Geometry: final body of the model. Coordinates: model frame, mm. Give positions to 0.01 mm unless a question says otherwise; leave off trailing zeros. Write each loop counter-clockwise with the first axis right and the second up, starting at its lowest first coordinate (ties: lowest second). Pieces come first, ordered by that corner, then holes.
Q1. Cut plane D-D on x = 14. Return the cut outline in (y, z) (3 decimals), plus the area to 3 significant figures.
Q2. Cut plane C-C on y = 15. Return the cut outline in (x, z) (3 decimals).
Q3. Line query: L1, parallel to X at y = 25, z = 0.8; L2, parallel to Y at x = 6, z = 1.7; L3, parallel to Z at x = 16.5, y = 17. Output: solid intervals per line, ascending.
Q4. Cut plane B-B on x = 6. Return the cut outline in (y, z).
Q5. Cut plane A-A on y = 5. Return the cut outline in (x, z).
Q6. Pin query (flat end, axial travel): pin 1 (4 mm diameter, centred on y = 20, z = -16, fed in from +X); pin 2 (10 mm diameter, centred on x = 16, z = -10, fed in from -Y) (3 decimals); pin 3 (2 mm diameter, centred on y = 14.5, z = -11.5, fed in from +X) (3 decimals); pin 4 (1 mm diameter, centred on x = 7.5, y = 22, fed in from -Z). Return the tip coordinate at first contact, or that it passes through.
Q7. Draft query along Y for faces 1 (the face through (23.5, 4.93, 1.52)), 2 (the face through (6.195, 23.513, 1.521)), 3 (the face through (16.305, 15.956, -23.91)), 4 (the face through (0, 15, 1)). Return one class per face: pulls with the +Y half, pulls with the -Y half, needs draft (parallel to the pull), parting line crosses it, or undercut.
```python
from build123d import *

# Parameters (mm, degrees)
SKETCH_1_W                      = 28
SKETCH_1_H                      = 30
EXTRUDE_1_DEPTH                 = 3
CUT_EXTRUDE_1_REACH             = 43.146
SKETCH_2_R                      = 1.5
CUT_EXTRUDE_1_DIRECTION_2_DEPTH = 42.146081223
SKETCH_3_R                      = 2.495
EXTRUDE_2_DEPTH                 = 48.5


with BuildPart() as part:
    # 草图1 → 凸台-拉伸1 (new body)
    with BuildSketch(Plane.XY):
        with Locations((14, 15)):
            Rectangle(SKETCH_1_W, SKETCH_1_H)
    extrude(amount=EXTRUDE_1_DEPTH)

    # 草图2 → 切除-拉伸1 (cut, up to next)
    with BuildSketch(Plane.XY.offset(3), mode=Mode.PRIVATE) as cut_extrude_1_sk1:
        with Locations(Location((6, 25, 0), (0, 0, 180))):
            Circle(SKETCH_2_R)
    cut_extrude_1_tool1 = extrude(cut_extrude_1_sk1.sketch, amount=-CUT_EXTRUDE_1_REACH, mode=Mode.PRIVATE) & part.part
    # 草图2 → 切除-拉伸1 (cut, up to next)
    with BuildSketch(Plane.XY.offset(3), mode=Mode.PRIVATE) as cut_extrude_1_sk2:
        with Locations(Location((22, 25, 0), (0, 0, 180))):
            Circle(SKETCH_2_R)
    cut_extrude_1_tool2 = extrude(cut_extrude_1_sk2.sketch, amount=-CUT_EXTRUDE_1_REACH, mode=Mode.PRIVATE) & part.part
    # 草图2 → 切除-拉伸1 (cut, up to next)
    with BuildSketch(Plane.XY.offset(3), mode=Mode.PRIVATE) as cut_extrude_1_sk3:
        with Locations(Location((22, 5, 0), (0, 0, 180))):
            Circle(SKETCH_2_R)
    cut_extrude_1_tool3 = extrude(cut_extrude_1_sk3.sketch, amount=-CUT_EXTRUDE_1_REACH, mode=Mode.PRIVATE) & part.part
    # 草图2 → 切除-拉伸1 (cut, up to next)
    with BuildSketch(Plane.XY.offset(3), mode=Mode.PRIVATE) as cut_extrude_1_sk4:
        with Locations(Location((6, 5, 0), (0, 0, 180))):
            Circle(SKETCH_2_R)
    cut_extrude_1_tool4 = extrude(cut_extrude_1_sk4.sketch, amount=-CUT_EXTRUDE_1_REACH, mode=Mode.PRIVATE) & part.part
    add(cut_extrude_1_tool1.solids().sort_by_distance((6, 25, 3))[0], mode=Mode.SUBTRACT)
    add(cut_extrude_1_tool2.solids().sort_by_distance((22, 25, 3))[0], mode=Mode.SUBTRACT)
    add(cut_extrude_1_tool3.solids().sort_by_distance((22, 5, 3))[0], mode=Mode.SUBTRACT)
    add(cut_extrude_1_tool4.solids().sort_by_distance((6, 5, 3))[0], mode=Mode.SUBTRACT)

    # 草图2 → 切除-拉伸1 direction 2 (cut)
    with BuildSketch(Plane.XY.offset(3)):
        with Locations(Location((6, 25, 0), (0, 0, 180))):
            Circle(SKETCH_2_R)
        with Locations(Location((22, 25, 0), (0, 0, 180))):
            Circle(SKETCH_2_R)
        with Locations(Location((22, 5, 0), (0, 0, 180))):
            Circle(SKETCH_2_R)
        with Locations(Location((6, 5, 0), (0, 0, 180))):
            Circle(SKETCH_2_R)
    extrude(amount=CUT_EXTRUDE_1_DIRECTION_2_DEPTH, mode=Mode.SUBTRACT)

    # 草图3 → 凸台-拉伸2 (add)
    with BuildSketch(Plane(origin=(0, 0, 0), x_dir=(-1, 0, 0), z_dir=(0, 0, -1))):
        with Locations(Location((-14, 15, 0), (0, 0, 180))):
            Circle(SKETCH_3_R)
    extrude(amount=EXTRUDE_2_DEPTH)


solid = part.part
```
Data:
1. outline: (0, 0) - (12.505, 0) - (12.505, -48.5) - (17.495, -48.5) - (17.495, 0) - (30, 0) - (30, 3) - (0, 3) - close
1. area: 332 mm2
2. outline: (0, 0) - (11.505, 0) - (11.505, -48.5) - (16.495, -48.5) - (16.495, 0) - (28, 0) - (28, 3) - (0, 3) - close
3. L1: x = 0 to 4.5, 7.5 to 20.5, 23.5 to 28
3. L2: y = 0 to 3.5, 6.5 to 23.5, 26.5 to 30
3. L3: z = 0 to 3
4. outline: (0, 0) - (3.5, 0) - (3.5, 3) - (0, 3) - close; (6.5, 0) - (23.5, 0) - (23.5, 3) - (6.5, 3) - close; (26.5, 0) - (30, 0) - (30, 3) - (26.5, 3) - close
5. outline: (0, 0) - (4.5, 0) - (4.5, 3) - (0, 3) - close; (7.5, 0) - (20.5, 0) - (20.5, 3) - (7.5, 3) - close; (23.5, 0) - (28, 0) - (28, 3) - (23.5, 3) - close
6. pin 1: passes through
6. pin 2: stops at y = 12.505
6. pin 3: stops at x = 16.495
6. pin 4: stops at z = 0
7. face 1: undercut
7. face 2: undercut
7. face 3: parting line crosses it
7. face 4: needs draft
